Here's the drawing with two shaded views (mm, measured from the low corner). I have some questions. A direction names the side the tool comes from. Round coordinates to 2 decimals unless told otherwise and drop trailing zeros. Order: outer loops, then holes, each group sorted by start corner. A loop starts at its lowest first (then second) coordinate and runs counter-clockwise, first axis right, second up. Notation, with made-up numbers: M 65,12.5 L 98,12.5 A16 ccw 98,42.5 Z; hole C 9,26.5 d9. An arc over 180 degrees is marked long. One line per question, with ' | ' between items.
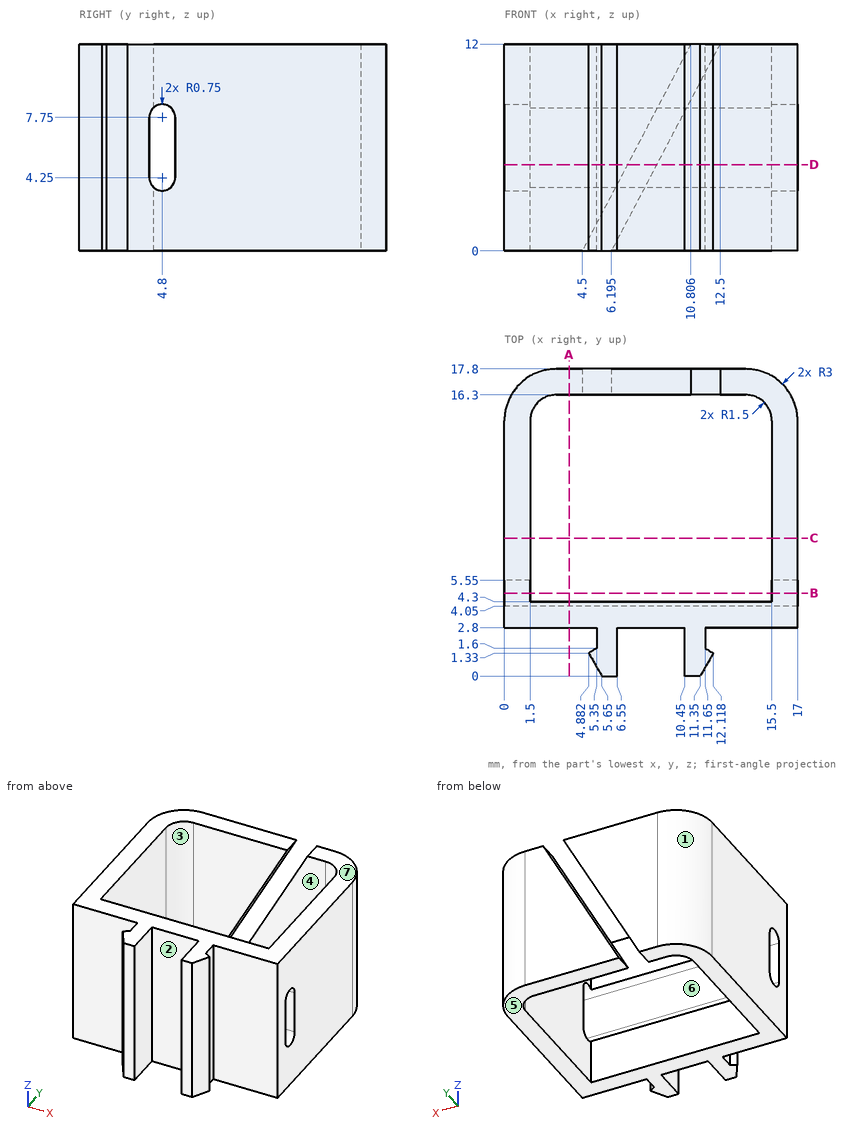
(1) If we section it at D-D on z = 5: State how many separate pieces and enclosed holes the cut face has.
Final values:
separate pieces: 3 | enclosed holes: 0
(2) If we section it at B-B on y = 4.8: Please give me the cut outline in (x, z), plus the area to 3 significant figures.
Final values:
outline: M 0,0 L 1.5,0 L 1.5,3.5 L 0,3.5 Z; M 0,8.5 L 1.5,8.5 L 1.5,12 L 0,12 Z; M 15.5,0 L 17,0 L 17,3.5 L 15.5,3.5 Z; M 15.5,8.5 L 17,8.5 L 17,12 L 15.5,12 Z | area: 21.0 mm^2
(3) Thinking about a two-plate mould opening in Z: for the marked faces 4, 5, 6 and 7, which applies, released by +Z, released by -Z, zero draft, split by the parting line, or undercut?
Final values:
face 4: zero draft | face 5: released by -Z | face 6: undercut | face 7: released by +Z
(4) If we section it at C-C on y = 8: Please give me the cut outline in (x, z).
Final values:
outline: M 0,0 L 1.5,0 L 1.5,12 L 0,12 Z; M 15.5,0 L 17,0 L 17,12 L 15.5,12 Z
(5) Will these pins go through, and if not, where does the flat tip stop? pin 1 Ø0.6 at (y, z) = (2, 8) entering from -X; pin 2 Ø1.5 at (x, z) = (13.5, 5) entering from -Y; pin 3 Ø0.8 at (y, z) = (1.5, 3.5) entering from -X; pin 4 Ø1.5 at (x, y) = (10.5, 5.5) entering from +Z.
Final values:
pin 1: x = 5.35 | pin 2: y = 2.8 | pin 3: x = 4.88 | pin 4: through
(6) Please list where these lines run through material, in increasing order: probe 1 along Y at (x, z) = (14, 1.5); probe 2 along X at (y, z) = (11.25, 1); probe 3 along Y at (x, z) = (5, 1.75) (1 decimal). Write a range as [from, to].
Final values:
probe 1: [2.8, 4.3], [16.3, 17.8] | probe 2: [0, 1.5], [15.5, 17] | probe 3: [1.1, 1.4], [2.8, 4.3], [16.3, 17.8]
(7) On a 3-axis mill with a long thin cutter (end or side, diameter ignored), from which of +Z, -Z, +X, -X, +Y, -Y can I reach the whole of each face in a straight line? I mean the marked faces 1, 2 and 3. Say none if no direction works.
Final values:
face 1: +Z, -Z, -X, +Y | face 2: +Z, -Z, -Y | face 3: +Z, -Z
(8) If we section it at A-A on x = 3.75: Please give me the cut outline in (y, z).
Final values:
outline: M 2.8,0 L 4.3,0 L 4.3,3.69 A0.75 cw 4.05,4.25 L 4.05,7.75 A0.75 cw 4.3,8.31 L 4.3,12 L 2.8,12 Z; M 16.3,0 L 17.8,0 L 17.8,12 L 16.3,12 Z
